```python
from build123d import *

# Parameters (mm, degrees)
SKETCH_1_W          = 140
SKETCH_1_H          = 149
EXTRUDE_1_DEPTH     = 2
EXTRUDE_2_DEPTH     = 2
FILLET_1_R          = 2
SKETCH_4_R          = 1.525
CUT_EXTRUDE_1_DEPTH = 2
CUT_EXTRUDE_3_DEPTH = 2
CUT_EXTRUDE_4_DEPTH = 2
FILLET_3_R          = 1.5
SKETCH_7_R          = 3.8
CUT_EXTRUDE_5_DEPTH = 22
CUT_EXTRUDE_START   = -22
CUT_EXTRUDE_6_DEPTH = 22
FILLET_4_R          = 1.1


with BuildPart() as part:
    # 草图1 → 凸台-拉伸1 (new body)
    with BuildSketch(Plane.XY):
        Rectangle(SKETCH_1_W, SKETCH_1_H)
    extrude(amount=EXTRUDE_1_DEPTH)

    # 草图2 → 凸台-拉伸2 (add)
    with BuildSketch(Plane.XY.offset(2)):
        with BuildLine():
            Line((-70, -74.5), (-4.275674814, -98.979595153))
            ThreePointArc((-4.275674814, -98.979595153), (0, -99.75), (4.275674814, -98.979595153))
            Line((4.275674814, -98.979595153), (70, -74.5))
            Line((70, -74.5), (-70, -74.5))
        make_face()
    extrude(amount=-EXTRUDE_2_DEPTH)

    # 圆角1
    fillet_1_edges = [part.edges().sort_by_distance(p)[0] for p in [
        (70, -74.5, 1),
        (-70, -74.5, 1),
        (-70, 74.5, 1),
        (70, 74.5, 1),
    ]]
    fillet(fillet_1_edges, radius=FILLET_1_R)

    # 草图4 → 切除-拉伸1 (cut)
    with BuildSketch(Plane(origin=(0, 0, 0), x_dir=(-1, 0, 0), z_dir=(0, 0, -1))):
        with Locations((8.5, -87.5)):
            Circle(SKETCH_4_R)
        with Locations((0, -96)):
            Circle(SKETCH_4_R)
        with Locations((-8.5, -87.5)):
            Circle(SKETCH_4_R)
        with Locations((0, -79)):
            Circle(SKETCH_4_R)
    extrude(amount=-CUT_EXTRUDE_1_DEPTH, mode=Mode.SUBTRACT)

    # 草图5 → 切除-拉伸3 (cut)
    with BuildSketch(Plane(origin=(0, 0, 0), x_dir=(-1, 0, 0), z_dir=(0, 0, -1))):
        Polygon((62, -44.439423724), (37.324827016, -72), (62, -72), align=None)
        Polygon((62, -17.454158494), (13.164733958, -72), (31.955917448, -72), (62, -38.442698117), align=None)
        Polygon((62, 9.531106736), (2, -57.485022296), (2, -72), (7.79582439, -72), (62, -11.457432887), align=None)
        Polygon((62, 36.516371966), (2, -30.499757066), (2, -51.488296689), (62, 15.527832343), align=None)
        Polygon((62, 63.501637197), (2, -3.514491836), (2, -24.503031459), (62, 42.513097573), align=None)
        Polygon((40.524361726, 66.5), (2, 23.470773395), (2, 2.482233771), (59.315545216, 66.5), align=None)
        Polygon((16.364268668, 66.5), (2, 50.456038625), (2, 29.467499001), (35.155452158, 66.5), align=None)
    cut_extrude_3 = extrude(amount=-CUT_EXTRUDE_3_DEPTH, mode=Mode.SUBTRACT)

    # 镜向1: 切除-拉伸3 across plane
    add(cut_extrude_3.mirror(Plane(origin=(0, 0, 0), x_dir=(0, 0, 1), z_dir=(1, 0, 0))), mode=Mode.SUBTRACT)

    # 草图6 → 切除-拉伸4 (cut)
    with BuildSketch(Plane.XY.offset(2)):
        Polygon((-10.9953591, 66.5), (10.9953591, 66.5), (0, 54.218893264), align=None)
    extrude(amount=-CUT_EXTRUDE_4_DEPTH, mode=Mode.SUBTRACT)

    # 圆角3
    fillet_3_edges = [part.edges().sort_by_distance(p)[0] for p in [
        (-2, -30.499757066, 1),
        (-62, 36.516371966, 1),
        (-62, 15.527832343, 1),
        (-2, -51.488296689, 1),
        (-2, -3.514491836, 1),
        (-62, 63.501637197, 1),
        (-62, 42.513097573, 1),
        (-2, -24.503031459, 1),
        (-62, -38.442698117, 1),
        (-31.955917448, -72, 1),
        (-13.164733958, -72, 1),
        (-62, -17.454158494, 1),
        (-2, -57.485022296, 1),
        (-62, 9.531106736, 1),
        (-62, -11.457432887, 1),
        (-7.79582439, -72, 1),
        (-2, -72, 1),
        (-2, 50.456038625, 1),
        (-16.364268668, 66.5, 1),
        (-35.155452158, 66.5, 1),
        (-2, 29.467499001, 1),
        (-2, 23.470773395, 1),
        (-40.524361726, 66.5, 1),
        (-59.315545216, 66.5, 1),
        (-2, 2.482233771, 1),
        (-62, -44.439423724, 1),
        (-62, -72, 1),
        (-37.324827016, -72, 1),
        (62, 15.527832343, 1),
        (2, -51.488296689, 1),
        (2, -30.499757066, 1),
        (62, 36.516371966, 1),
        (62, 42.513097573, 1),
        (2, -24.503031459, 1),
        (2, -3.514491836, 1),
        (62, 63.501637197, 1),
        (13.164733958, -72, 1),
        (62, -17.454158494, 1),
        (62, -38.442698117, 1),
        (31.955917448, -72, 1),
        (62, -11.457432887, 1),
        (7.79582439, -72, 1),
        (2, -72, 1),
        (2, -57.485022296, 1),
        (62, 9.531106736, 1),
        (35.155452158, 66.5, 1),
        (2, 29.467499001, 1),
        (2, 50.456038625, 1),
        (16.364268668, 66.5, 1),
        (59.315545216, 66.5, 1),
        (2, 2.482233771, 1),
        (2, 23.470773395, 1),
        (40.524361726, 66.5, 1),
        (37.324827016, -72, 1),
        (62, -44.439423724, 1),
        (62, -72, 1),
        (10.9953591, 66.5, 1),
        (-10.9953591, 66.5, 1),
        (0, 54.218893264, 1),
    ]]
    fillet(fillet_3_edges, radius=FILLET_3_R)

    # 草图7 → 切除-拉伸5 (cut)
    with BuildSketch(Plane(origin=(0, 0, 0), x_dir=(-1, 0, 0), z_dir=(0, 0, -1))):
        with Locations((0, -87.5)):
            Circle(SKETCH_7_R)
    extrude(amount=-CUT_EXTRUDE_5_DEPTH, mode=Mode.SUBTRACT)

    # 草图8 → 切除-拉伸6 (cut)
    with BuildSketch(Plane(origin=(0, 0, 0), x_dir=(-1, 0, 0), z_dir=(0, 0, -1)).offset(CUT_EXTRUDE_START)):
        with BuildLine():
            Line((48.962621857, -77), (11.783719365, -90.847604805))
            ThreePointArc((11.783719365, -90.847604805), (11.392195972, -82.996626716), (6.309714732, -77))
            Line((6.309714732, -77), (48.962621857, -77))
        make_face()
    cut_extrude_6 = extrude(amount=CUT_EXTRUDE_6_DEPTH, mode=Mode.SUBTRACT)

    # 镜向2: 切除-拉伸6 across plane
    add(cut_extrude_6.mirror(Plane(origin=(0, 0, 0), x_dir=(0, 0, 1), z_dir=(1, 0, 0))), mode=Mode.SUBTRACT)

    # 圆角4
    fillet_4_edges = [part.edges().sort_by_distance(p)[0] for p in [
        (-6.309714732, -77, 1),
        (-48.962621857, -77, 1),
        (-11.783719365, -90.847604805, 1),
        (48.962621857, -77, 1),
        (6.309714732, -77, 1),
        (11.783719365, -90.847604805, 1),
    ]]
    fillet(fillet_4_edges, radius=FILLET_4_R)


solid = part.part
```
CAD build for the part. Positions are in the model's coordinates, mm. A direction names the side the tool comes from. Coordinates: 2 decimals unless noted, no trailing zeros. Order: outer loops, then holes, each group sorted by start corner. A loop starts at its lowest first (then second) coordinate and runs counter-clockwise, first axis right, second up. Notation, with made-up numbers: (-12.5, -23) -> (30.5, -23) arc R28 cw to (30.5, 2) -> close; hole circle Ø5 at (-1, 83). An arc over 180 degrees is marked (long way). Use one line per item in the form item = value. Start each with the question number.
1) Drop flat-ended pins along their axis: pin 1 (0.6 mm diameter, centred on x = 22, z = 0.5, fed in from -Y); pin 2 (1 mm diameter, centred on x = -23, z = 1, fed in from -Y); pin 3 (1 mm diameter, centred on x = 22.5, z = 0.5, fed in from -Y). Give the stop position or say it passes through.
2) Pull direction Y, two halves, no side cores. Call faces 1 (the flat face through (-36.938, -86.814, 1.014)), 2 (the flat face through (0, -12, 0)), 3 (the flat face through (31.28, 29.19, 0.99)): +Y half, -Y half, draft (parallel to the pull), parting line (faces both ways), or undercut.
3) Tool access for faces 4 (the flat face through (-31.28, 29.19, 0.99)), 5 (the flat face through (36.04, -87.15, 1.01)): list every direction of +Z, -Z, +X, -X, +Y, -Y with a clear straight run to the whole face (end or side of a thin tool).
4) Drill centre line: L1, parallel to Y at x = 64, z = 1.5. Where is it in solid material? Low to high. Write a range as [from, to].
5) Band-saw the part on B-B on z = 1.2. State how many separate pieces and enclosed holes the cut face has, then the cut area to 3 significant figures.
6) Band-saw the part on A-A on y = 0. Give the cut face in (x, z).
Entries:
q1.pin_1 = -92.49
q1.pin_2 = -92.19
q1.pin_3 = -92.38
q2.face_1 = -Y half
q2.face_2 = draft
q2.face_3 = undercut
q3.face_4 = +Z, -Z
q3.face_5 = +Z, -Z, +X, -Y
q4.L1 = [-76.73, 74.5]
q5.separate_pieces = 1
q5.enclosed_holes = 22
q5.area = 9,170 mm2
q6.outline = (-70, 0) -> (-62, 0) -> (-62, 2) -> (-70, 2) -> close; (-53.47, 0) -> (-48.1, 0) -> (-48.1, 2) -> (-53.47, 2) -> close; (-29.31, 0) -> (-23.94, 0) -> (-23.94, 2) -> (-29.31, 2) -> close; (-5.15, 0) -> (5.15, 0) -> (5.15, 2) -> (-5.15, 2) -> close; (23.94, 0) -> (29.31, 0) -> (29.31, 2) -> (23.94, 2) -> close; (48.1, 0) -> (53.47, 0) -> (53.47, 2) -> (48.1, 2) -> close; (62, 0) -> (70, 0) -> (70, 2) -> (62, 2) -> close
